Design review of the part built by this model. Coordinates are the model's own, in mm. Round coordinates to 2 decimals unless told otherwise and drop trailing zeros. Loops run counter-clockwise (first coordinate to the right, second up) from the corner with the lowest first, then second, coordinate; pieces in that order, holes last. Notation, with made-up numbers: (-11.75, -36.75) - (3.25, -36.75) arc R25 cw to (3.25, -2.75) - close; hole circle Ø4 at (12, -13.5). An arc over 180 degrees is marked (long way). One line per question, with ' | ' between items. Start each with the question number.
from build123d import *

# Parameters (mm, degrees)
BOSS_EXTRUDE1_DEPTH                          = 2
CUT_EXTRUDE1_REACH                           = 103.772
SKETCH3_R                                    = 1.75
CHAMFER1_SIZE                                = 3
FILLET1_R                                    = 5
CUT_EXTRUDE2_REACH                           = 103.772
SKETCH4_R                                    = 1.75
CUT_EXTRUDE3_REACH                           = 103.772
SKETCH5_R                                    = 1.75
CSK_FOR_M3_HEX_SOCKET_COUNTERSUNK_HE_2_COUNT = 2
CSK_FOR_M3_HEX_SOCKET_COUNTERSUNK_HE_2_PITCH = 37.443290454
CSK_FOR_M3_HEX_SOCKET_COUNTERSUNK_HE_3_COUNT = 2
CSK_FOR_M3_HEX_SOCKET_COUNTERSUNK_HE_3_PITCH = 37.443290454


with BuildPart() as part:
    # Sketch2 → Boss-Extrude1 (new body)
    with BuildSketch(Plane(origin=(0, 0, 0), x_dir=(1, 0, 0), z_dir=(0, 1, 0))):
        Polygon((-58.355339059, 0), (58.355339059, 0), (58.355339059, 49.171572875), (24.171572875, 83.355339059), (-24.171572875, 83.355339059), (-58.355339059, 49.171572875), align=None)
    extrude(amount=BOSS_EXTRUDE1_DEPTH)

    # Sketch3 → Cut-Extrude1 (cut, up to next)
    with BuildSketch(Plane.XZ, mode=Mode.PRIVATE) as cut_extrude1_sk1:
        with Locations(Location((-43.355339059, -24.315188388, 0), (0, 0, 270))):
            Circle(SKETCH3_R)
    cut_extrude1_tool1 = extrude(cut_extrude1_sk1.sketch, amount=-CUT_EXTRUDE1_REACH, mode=Mode.PRIVATE) & part.part
    # Sketch3 → Cut-Extrude1 (cut, up to next)
    with BuildSketch(Plane.XZ, mode=Mode.PRIVATE) as cut_extrude1_sk2:
        with Locations(Location((-30.656854249, -55.656854249, 0), (0, 0, 270))):
            Circle(SKETCH3_R)
    cut_extrude1_tool2 = extrude(cut_extrude1_sk2.sketch, amount=-CUT_EXTRUDE1_REACH, mode=Mode.PRIVATE) & part.part
    # Sketch3 → Cut-Extrude1 (cut, up to next)
    with BuildSketch(Plane.XZ, mode=Mode.PRIVATE) as cut_extrude1_sk3:
        with Locations(Location((0, -68.355339059, 0), (0, 0, 270))):
            Circle(SKETCH3_R)
    cut_extrude1_tool3 = extrude(cut_extrude1_sk3.sketch, amount=-CUT_EXTRUDE1_REACH, mode=Mode.PRIVATE) & part.part
    # Sketch3 → Cut-Extrude1 (cut, up to next)
    with BuildSketch(Plane.XZ, mode=Mode.PRIVATE) as cut_extrude1_sk4:
        with Locations(Location((30.656854249, -55.656854249, 0), (0, 0, 270))):
            Circle(SKETCH3_R)
    cut_extrude1_tool4 = extrude(cut_extrude1_sk4.sketch, amount=-CUT_EXTRUDE1_REACH, mode=Mode.PRIVATE) & part.part
    # Sketch3 → Cut-Extrude1 (cut, up to next)
    with BuildSketch(Plane.XZ, mode=Mode.PRIVATE) as cut_extrude1_sk5:
        with Locations(Location((43.355339059, -24.315188388, 0), (0, 0, 270))):
            Circle(SKETCH3_R)
    cut_extrude1_tool5 = extrude(cut_extrude1_sk5.sketch, amount=-CUT_EXTRUDE1_REACH, mode=Mode.PRIVATE) & part.part
    add(cut_extrude1_tool1.solids().sort_by_distance((-43.355339, 0, -24.315188))[0], mode=Mode.SUBTRACT)
    add(cut_extrude1_tool2.solids().sort_by_distance((-30.656854, 0, -55.656854))[0], mode=Mode.SUBTRACT)
    add(cut_extrude1_tool3.solids().sort_by_distance((0, 0, -68.355339))[0], mode=Mode.SUBTRACT)
    add(cut_extrude1_tool4.solids().sort_by_distance((30.656854, 0, -55.656854))[0], mode=Mode.SUBTRACT)
    add(cut_extrude1_tool5.solids().sort_by_distance((43.355339, 0, -24.315188))[0], mode=Mode.SUBTRACT)

    # Chamfer1
    chamfer1_edges = [part.edges().sort_by_distance(p)[0] for p in [
        (58.355339059, 1, 0),
        (-58.355339059, 1, 0),
    ]]
    chamfer(chamfer1_edges, length=CHAMFER1_SIZE)

    # Fillet1
    fillet1_edges = [part.edges().sort_by_distance(p)[0] for p in [
        (-58.355339059, 1, -49.171572875),
        (-24.171572875, 1, -83.355339059),
        (24.171572875, 1, -83.355339059),
        (58.355339059, 1, -49.171572875),
    ]]
    fillet(fillet1_edges, radius=FILLET1_R)

    # Sketch4 → Cut-Extrude2 (cut, up to next)
    with BuildSketch(Plane(origin=(0, 2, 0), x_dir=(1, 0, 0), z_dir=(0, 1, 0)), mode=Mode.PRIVATE) as cut_extrude2_sk1:
        with Locations(Location((-20, 45, 0), (0, 0, 270))):
            Circle(SKETCH4_R)
    cut_extrude2_tool1 = extrude(cut_extrude2_sk1.sketch, amount=-CUT_EXTRUDE2_REACH, mode=Mode.PRIVATE) & part.part
    # Sketch4 → Cut-Extrude2 (cut, up to next)
    with BuildSketch(Plane(origin=(0, 2, 0), x_dir=(1, 0, 0), z_dir=(0, 1, 0)), mode=Mode.PRIVATE) as cut_extrude2_sk2:
        with Locations(Location((20, 5, 0), (0, 0, 270))):
            Circle(SKETCH4_R)
    cut_extrude2_tool2 = extrude(cut_extrude2_sk2.sketch, amount=-CUT_EXTRUDE2_REACH, mode=Mode.PRIVATE) & part.part
    add(cut_extrude2_tool1.solids().sort_by_distance((-20, 2, -45))[0], mode=Mode.SUBTRACT)
    add(cut_extrude2_tool2.solids().sort_by_distance((20, 2, -5))[0], mode=Mode.SUBTRACT)

    # Sketch5 → Cut-Extrude3 (cut, up to next)
    with BuildSketch(Plane(origin=(0, 2, 0), x_dir=(1, 0, 0), z_dir=(0, 1, 0)), mode=Mode.PRIVATE) as cut_extrude3_sk1:
        with Locations(Location((0, 37, 0), (0, 0, 270))):
            Circle(SKETCH5_R)
    cut_extrude3_tool1 = extrude(cut_extrude3_sk1.sketch, amount=-CUT_EXTRUDE3_REACH, mode=Mode.PRIVATE) & part.part
    # Sketch5 → Cut-Extrude3 (cut, up to next)
    with BuildSketch(Plane(origin=(0, 2, 0), x_dir=(1, 0, 0), z_dir=(0, 1, 0)), mode=Mode.PRIVATE) as cut_extrude3_sk2:
        with Locations(Location((-31, 16, 0), (0, 0, 270))):
            Circle(SKETCH5_R)
    cut_extrude3_tool2 = extrude(cut_extrude3_sk2.sketch, amount=-CUT_EXTRUDE3_REACH, mode=Mode.PRIVATE) & part.part
    # Sketch5 → Cut-Extrude3 (cut, up to next)
    with BuildSketch(Plane(origin=(0, 2, 0), x_dir=(1, 0, 0), z_dir=(0, 1, 0)), mode=Mode.PRIVATE) as cut_extrude3_sk3:
        with Locations(Location((31, 16, 0), (0, 0, 270))):
            Circle(SKETCH5_R)
    cut_extrude3_tool3 = extrude(cut_extrude3_sk3.sketch, amount=-CUT_EXTRUDE3_REACH, mode=Mode.PRIVATE) & part.part
    add(cut_extrude3_tool1.solids().sort_by_distance((0, 2, -37))[0], mode=Mode.SUBTRACT)
    add(cut_extrude3_tool2.solids().sort_by_distance((-31, 2, -16))[0], mode=Mode.SUBTRACT)
    add(cut_extrude3_tool3.solids().sort_by_distance((31, 2, -16))[0], mode=Mode.SUBTRACT)

    # Sketch6 → CSK for M3 Hex Socket Countersunk Head Screw1 (revolve, cut)
    with BuildSketch(Plane(origin=(0, 2, -37), x_dir=(0, 0, 1), z_dir=(1, 0, 0))):
        Polygon((0, 0), (0, 2), (1.7, 2), (1.7, 1.77), (3.47, 0), align=None)
    csk_for_m3_hex_socket_countersunk_head_s = revolve(axis=Axis((0, 8.35, -37), (0, -1, 0)), mode=Mode.SUBTRACT)

    # CSK for M3 Hex Socket Countersunk He 2: CSK for M3 Hex Socket Countersunk Head Screw1 ×2
    with Locations(*[Vector(-0.827918690488332, 0, 0.5608481451695153) * (i * CSK_FOR_M3_HEX_SOCKET_COUNTERSUNK_HE_2_PITCH) for i in range(1, CSK_FOR_M3_HEX_SOCKET_COUNTERSUNK_HE_2_COUNT)]):
        add(csk_for_m3_hex_socket_countersunk_head_s, mode=Mode.SUBTRACT)

    # CSK for M3 Hex Socket Countersunk He 3: CSK for M3 Hex Socket Countersunk Head Screw1 ×2
    with Locations(*[Vector(0.827918690488332, 0, 0.5608481451695153) * (i * CSK_FOR_M3_HEX_SOCKET_COUNTERSUNK_HE_3_PITCH) for i in range(1, CSK_FOR_M3_HEX_SOCKET_COUNTERSUNK_HE_3_COUNT)]):
        add(csk_for_m3_hex_socket_countersunk_head_s, mode=Mode.SUBTRACT)


solid = part.part
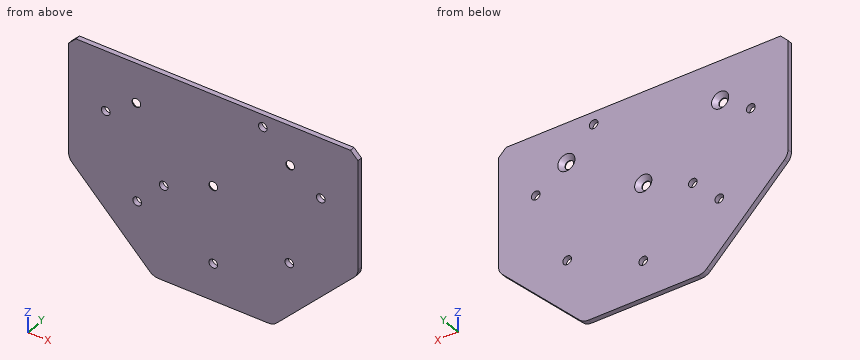
1. Take a section at C-C, the plane y = 1. Count the separate pieces of the cut face and the enclosed holes in it, then the cut area to 3 significant figures.
2. Take a section at B-B, the plane z = -16. Give the boundary of the cut face in (x, y).
3. Take a section at D-D, the plane x = -36. Give the boundary of the cut face in (y, z).
4. Take a section at A-A, the plane z = -45. Give the boundary of the cut face in (x, y), then the cut area to 3 significant figures.
5. To check wall thickness, follow line 1 along X through (y, z) = (0.1, -16); line 2 along Z through (x, y) = (-32, 0.2); line 3 along Z through (x, y) = (-31, 0.2). State the ranges of each line that lie inside material, in increasing order.
6. Clearance check with a flat-ended pin moving along its axis: P1, Ø1, axis at x = 31.5, y = 1.5, coming from the -Z side. State where the tip first meets the part, or that it passes through.
Answer list:
1) separate pieces: 1 | enclosed holes: 10 | area: 8,420 mm²
2) outline: (-58.36, 0) - (-32.75, 0) - (-32.75, 0.28) - (-34.47, 2) - (-58.36, 2) - close; (-29.25, 0) - (29.25, 0) - (29.25, 0.28) - (27.53, 2) - (-27.53, 2) - (-29.25, 0.28) - close; (32.75, 0) - (58.36, 0) - (58.36, 2) - (34.47, 2) - (32.75, 0.28) - close
3) outline: (0, -71.53) - (2, -71.53) - (2, 0) - (0, 0) - close
4) outline: (-58.36, 0) - (-21.75, 0) - (-21.75, 2) - (-58.36, 2) - close; (-18.25, 0) - (58.36, 0) - (58.36, 2) - (-18.25, 2) - close | area: 226 mm²
5) line 1: x = -58.36 to -32.75, -29.25 to 29.25, 32.75 to 58.36 | line 2: z = -75.53 to -56.78, -54.54 to -17.44, -14.56 to 0 | line 3: z = -76.53 to -57.37, -53.94 to -17.75, -14.25 to 0
6) P1: stops at z = -76.53
